```python
from build123d import *

# Parameters (mm, degrees)
F0_R     = 2.1
F1_DEPTH = 3
F2_R     = 5
F3_R     = 6.5
F4_DEPTH = 10
F5_R     = 1


with BuildPart() as f1:
    # F0 (on Top) → F1 (new body)
    with BuildSketch(Plane.XY):
        with BuildLine():
            ThreePointArc((-5.656854, -7), (-8.485281, 3), (0, 9))
            Line((0, 9), (-23.064781, 9))
            Line((-23.064781, 9), (-23.064781, -7))
            Line((-23.064781, -7), (-5.656854, -7))
        make_face()
        with Locations((-18, -2)):
            Circle(F0_R, mode=Mode.SUBTRACT)
        with BuildLine():
            ThreePointArc((0, -6), (-6, 0), (0, 6))
            Line((0, 6), (0, 9))
            ThreePointArc((0, 9), (-8.485281, 3), (-5.656854, -7))
            Line((-5.656854, -7), (0, -7))
            Line((0, -7), (0, -6))
        make_face()
        with BuildLine():
            ThreePointArc((0, 6), (4.242641, 4.242641), (6, 0))
            ThreePointArc((6, 0), (4.242641, -4.242641), (0, -6))
            Line((0, -6), (0, -7))
            Line((0, -7), (-5.656854, -7))
            ThreePointArc((-5.656854, -7), (3.87868, -8.12132), (9, 0))
            ThreePointArc((9, 0), (6.363961, 6.363961), (0, 9))
            Line((0, 9), (0, 6))
        make_face()
    extrude(amount=F1_DEPTH)

    # F2
    f2_edges = [f1.edges().sort_by_distance(p)[0] for p in [
        (-23.064781, 9, 1.5),
        (-23.064781, -7, 1.5),
    ]]
    fillet(f2_edges, radius=F2_R)

    # F3 (on face) → F4 (join)
    with BuildSketch(Plane.XY.offset(3)):
        with BuildLine():
            ThreePointArc((-5.656854, -7), (3.87868, -8.12132), (9, 0))
            ThreePointArc((9, 0), (6.363961, 6.363961), (0, 9))
            ThreePointArc((0, 9), (-8.485281, 3), (-5.656854, -7))
        make_face()
        Circle(F3_R, mode=Mode.SUBTRACT)
    extrude(amount=F4_DEPTH)

    # F5
    f5_edges = [f1.edges().sort_by_distance(p)[0] for p in [
        (0, -9, 13),
        (-6.5, 0, 13),
    ]]
    fillet(f5_edges, radius=F5_R)


solid = f1.part
```
Here's how the part is built. I have some questions about the finished solid (model axes, mm). A direction names the side the tool comes from. Coordinates: 2 decimals unless noted, no trailing zeros. Write each loop counter-clockwise with the first axis right and the second up, starting at its lowest first coordinate (ties: lowest second). Pieces come first, ordered by that corner, then holes. Notation, with made-up numbers: (63.25, 26) -> (80.25, 26) arc R22 ccw to (80.25, 38) -> close; hole circle Ø4 at (6.25, 34). An arc over 180 degrees is marked (long way). Use a Markdown table: item, result. Add a question column.
(1) Please list where these lines run through material, in increasing order: line 1 (Y direction, x = -18, z = 1.7); line 2 (Y direction, x = 0, z = 8.25); line 3 (Z direction, x = -11, y = 3.5).
(2) If we section it at A-A, the plane z = 5: Write out the boundary of the cut face in (x, y).
(3) If we section it at B-B, the plane y = -3: State how many separate pieces and enclosed holes the cut face has, and give its area (3 significant figures).
(4) For faces 4 (the cylindrical face through (-21.561, 7.574, 1.521)), 5 (the flat face through (-12, -7, 1)), 6 (the flat face through (2, -6, 3)), which set-ups out of +Z, -Z, +X, -X, +Y, -Y let a thin tool reach every point of the face, with its end or its side?
(5) I'm going to push flat-ended pins straight in: P1, Ø3, axis at x = -1, z = 11.5, coming from the -Y side; P2, Ø6, axis at x = -10.5, z = 2, coming from the -Y side; P3, Ø4, axis at y = 2, z = 10, coming from the -X side; P4, Ø8, axis at x = -16, y = 5, coming from the +Z side. Where does each tip first touch, or does it pass through?
(6) We'd pull the mould along X, two halves only. Please class faces 1 (the flat face through (6, -5, 13)), 2 (the cylindrical face through (-21.561, -5.574, 1.521)), 3 (the cylindrical face through (-5.158, -3.955, 7.437)): +X half, -X half, draft (parallel to the pull), parting line (faces both ways), or undercut.
Outcome:
| question | item | result |
|---|---|---|
| 1 | line 1 | y = -7 to -4.1, 0.1 to 9 |
| 1 | line 2 | y = -9 to -6.5, 6.5 to 9 |
| 1 | line 3 | z = 0 to 3 |
| 2 | outline | circle Ø18 at (0, 0); hole circle Ø13 at (0, 0) |
| 3 | separate pieces | 3 |
| 3 | enclosed holes | 0 |
| 3 | area | 106 mm^2 |
| 4 | face 4 | +Z, -Z, -X, +Y |
| 4 | face 5 | +Z, -Z, -X, -Y |
| 4 | face 6 | +Z |
| 5 | P1 | stops at y = -9 |
| 5 | P2 | stops at y = -7 |
| 5 | P3 | stops at x = -9 |
| 5 | P4 | stops at z = 3 |
| 6 | face 1 | draft |
| 6 | face 2 | -X half |
| 6 | face 3 | undercut |
